```python
from build123d import *

# Parameters (mm, degrees)
BOSS_EXTRUDE1_DEPTH = 6
SKETCH3_R           = 3.5
CUT_EXTRUDE2_DEPTH  = 4
SKETCH4_R           = 2
CUT_EXTRUDE3_DEPTH  = 6
SKETCH6_R           = 3.6
CUT_EXTRUDE4_DEPTH  = 6
CUT_EXTRUDE6_START  = -6
SKETCH10_R          = 1.5
CUT_EXTRUDE6_DEPTH  = 4


with BuildPart() as part:
    # Sketch1 → Boss-Extrude1 (new body)
    with BuildSketch(Plane.XY):
        Polygon((-37, 30), (-40, 30), (-40, 27), (-40, -27), (-40, -30), (-37, -30), (37, -30), (44, -30), (44, -27), (44, 27), (44, 30), (37, 30), align=None)
    extrude(amount=BOSS_EXTRUDE1_DEPTH)

    # Sketch3 → Cut-Extrude2 (cut)
    with BuildSketch(Plane.XY.offset(6)):
        with Locations((-36, 26)):
            Circle(SKETCH3_R)
        with Locations((40, 26)):
            Circle(SKETCH3_R)
        with Locations((40, -26)):
            Circle(SKETCH3_R)
        with Locations((-36, -26)):
            Circle(SKETCH3_R)
    extrude(amount=-CUT_EXTRUDE2_DEPTH, mode=Mode.SUBTRACT)

    # Sketch4 → Cut-Extrude3 (cut)
    with BuildSketch(Plane.XY.offset(6)):
        with Locations((-36, 26)):
            Circle(SKETCH4_R)
        with Locations((40, 26)):
            Circle(SKETCH4_R)
        with Locations((40, -26)):
            Circle(SKETCH4_R)
        with Locations((-36, -26)):
            Circle(SKETCH4_R)
    extrude(amount=-CUT_EXTRUDE3_DEPTH, mode=Mode.SUBTRACT)

    # Sketch6 → Cut-Extrude4 (cut)
    with BuildSketch(Plane(origin=(0, 0, 0), x_dir=(-1, 0, 0), z_dir=(0, 0, -1))):
        with Locations((-2, -20.5)):
            Circle(SKETCH6_R)
        Polygon((30.5, -8), (-34.5, -8), (-38, -8), (-38, 16), (-2, 16), (34, 16), (34, -8), align=None)
    extrude(amount=-CUT_EXTRUDE4_DEPTH, mode=Mode.SUBTRACT)

    # Sketch10 → Cut-Extrude6 (cut)
    with BuildSketch(Plane.XY.offset(6).offset(CUT_EXTRUDE6_START)):
        with Locations((-36, 20)):
            Circle(SKETCH10_R)
        with Locations((40, 20)):
            Circle(SKETCH10_R)
        with Locations((40, -12)):
            Circle(SKETCH10_R)
        with Locations((-36, -12)):
            Circle(SKETCH10_R)
    extrude(amount=CUT_EXTRUDE6_DEPTH, mode=Mode.SUBTRACT)


solid = part.part
```
For this review, take the finished solid that the model builds, in its own axes (mm). A direction names the side the tool comes from. Coordinates: 2 decimals unless noted, no trailing zeros. Write each loop counter-clockwise with the first axis right and the second up, starting at its lowest first coordinate (ties: lowest second). Pieces come first, ordered by that corner, then holes.
(1) The part is to be moulded in two halves that separate along Y. For faces 1 (the face through (40, 20, 4)), 2 (the face through (3, 30, 3)), 3 (the face through (44, 0, 3)), 4 (the face through (-34, 4, 3)), say which applies: +Y half, -Y half, draft (parallel to the pull), parting line (faces both ways), or undercut.
(2) Wall thickness on probe 1 along Y at (x, z) = (40, 0.95); probe 2 along Y at (x, z) = (35, 1.25); probe 3 along X at (y, z) = (26.5, 1.3): over which ranges is each line inside the solid? List them lowest first.
(3) For pin 1 Ø2.5 at (x, y) = (-36, 20) entering from -Z; pin 2 Ø1.5 at (x, y) = (28.5, -5.5) entering from +Z; pin 3 Ø4.5 at (x, y) = (40, -26) entering from +Z, all flat-tipped, find the tip position at first contact; note any pin that passes through.
(4) Add section D-D on y = 2. Give the boundary of the cut face in (x, z).
(5) Add section C-C on y = 26. Give the boundary of the cut face in (x, z).
(6) Add section A-A on x = -36. Give the boundary of the cut face in (y, z).
(7) Tool access review of faces 5 (the face through (38, 4, 3)), 6 (the face through (42, 24, 2)), 7 (the face through (38.5, -11.93, 1.97)): name each direction out of +Z, -Z, +X, -X, +Y, -Y from which nothing blocks a thin tool from reaching the whole face with its end or side.
(8) Add section B-B on z = 2.9. Count the separate pieces of the cut face and the enclosed holes in it, then the cut area to 3 significant figures.
Answer sheet:
1. face 1: undercut
1. face 2: +Y half
1. face 3: draft
1. face 4: undercut
2. probe 1: y = -30 to -28, -24 to -13.5, -10.5 to 18.5, 21.5 to 24, 28 to 30
2. probe 2: y = -30 to -8, 16 to 30
2. probe 3: x = -40 to -37.94, -34.06 to 38.06, 41.94 to 44
3. pin 1: stops at z = 4
3. pin 2: passes through
3. pin 3: stops at z = 2
4. outline: (-40, 0) - (-34, 0) - (-34, 6) - (-40, 6) - close; (38, 0) - (44, 0) - (44, 6) - (38, 6) - close
5. outline: (-40, 0) - (-38, 0) - (-38, 2) - (-39.5, 2) - (-39.5, 6) - (-40, 6) - close; (-34, 0) - (38, 0) - (38, 2) - (36.5, 2) - (36.5, 6) - (-32.5, 6) - (-32.5, 2) - (-34, 2) - close; (42, 0) - (44, 0) - (44, 6) - (43.5, 6) - (43.5, 2) - (42, 2) - close
6. outline: (-30, 0) - (-28, 0) - (-28, 2) - (-29.5, 2) - (-29.5, 6) - (-30, 6) - close; (-24, 0) - (-13.5, 0) - (-13.5, 4) - (-10.5, 4) - (-10.5, 0) - (18.5, 0) - (18.5, 4) - (21.5, 4) - (21.5, 0) - (24, 0) - (24, 2) - (22.5, 2) - (22.5, 6) - (-22.5, 6) - (-22.5, 2) - (-24, 2) - close; (28, 0) - (30, 0) - (30, 6) - (29.5, 6) - (29.5, 2) - (28, 2) - close
7. face 5: +Z, -Z
7. face 6: +Z
7. face 7: -Z
8. separate pieces: 1
8. enclosed holes: 10
8. area: 3,090 mm2
